Part model, mm, in its own coordinate system. Face numbers are marked on the shaded views. A direction names the side the tool comes from. Coordinates: 2 decimals unless noted, no trailing zeros. Loops run counter-clockwise (first coordinate to the right, second up) from the corner with the lowest first, then second, coordinate; pieces in that order, holes last. Notation, with made-up numbers: (9.25, 48) -> (21.25, 48) arc R13 cw to (21.25, 59) -> close; hole circle Ø8 at (19, 68). An arc over 180 degrees is marked (long way). Use one line per item in the form item = value. Start each with the question number.
(1) Drill centre lines: L1, parallel to X at y = 39, z = 5.25; L2, parallel to Y at x = 0.25, z = 2.5; L3, parallel to Z at x = 8.25, y = -20.5. Where is each one in solid material? Low to high. Write a range as [from, to].
(2) Pin check, flat tips, straight feed: P1, Ø5, axis at x = -9.39, y = 0.55, coming from the +Z side; P2, Ø5, axis at x = 1.5, z = 11.5, coming from the -Y side; P3, Ø5, axis at x = -9.5, z = 17.5, coming from the -Y side; P4, Ø3, axis at x = 6.91, z = 10, coming from the +Y side. Stop position of each tip, or through.
(3) Band-saw the part on B-B on y = 15. Give the cut face in (x, z), then the cut area to 3 significant figures.
(4) Band-saw the part on A-A on y = -31.5. Give the cut face in (x, z) (3 decimals), then the cut area to 3 significant figures.
(5) 3-axis set-ups, long thin cutter, end or side, ignore diameter. For the marked faces 1 and 2: which of +Z, -Z, +X, -X, +Y, -Y reach the whole face in a straight line?
(6) Band-saw the part on C-C on z = 10.75. Count the separate pieces of the cut face and the enclosed holes in it, then the cut area to 3 significant figures.
(7) Mould opens along X. For the marked faces 3, 4 and 5 say: +X half, -X half, draft (parallel to the pull), parting line (faces both ways), or undercut.
```python
from build123d import *

# Parameters (mm, degrees)
ESQUISSE1_W                  = 22.45
ESQUISSE1_H                  = 85
BOSS_EXTRU_1_DEPTH           = 4
ESQUISSE2_R                  = 3
ENL_V_MAT_EXTRU_1_DEPTH      = 4
ESQUISSE3_R                  = 1.6
ENL_V_MAT_EXTRU_2_DEPTH      = 4
ESQUISSE4_W                  = 3
ESQUISSE4_H                  = 38.437504141
BOSS_EXTRU_2_DEPTH           = 20
CONG_1_R                     = 2
ESQUISSE7_W                  = 27.642878523
ESQUISSE7_H                  = 19.995510754
BOSS_EXTRU_3_DEPTH           = 2
BOSS_EXTRU_3_TAPER           = 1
BOSS_EXTRU_3_OTHER_WAY_DEPTH = 1
BOSS_EXTRU_3_OTHER_WAY_TAPER = 1
ESQUISSE8_R                  = 1.7
ENL_V_MAT_EXTRU_3_DEPTH      = 58


with BuildPart() as part:
    # Esquisse1 → Boss.-Extru.1 (new body)
    with BuildSketch(Plane.XY):
        Rectangle(ESQUISSE1_W, ESQUISSE1_H)
    extrude(amount=BOSS_EXTRU_1_DEPTH)

    # Esquisse2 → Enlèv. mat.-Extru.1 (cut)
    with BuildSketch(Plane.XY):
        with Locations((0, -31.5)):
            Circle(ESQUISSE2_R)
    extrude(amount=ENL_V_MAT_EXTRU_1_DEPTH, mode=Mode.SUBTRACT)

    # Esquisse3 → Enlèv. mat.-Extru.2 (cut)
    with BuildSketch(Plane.XY):
        with Locations((-9.391474789, 0.549780329)):
            Circle(ESQUISSE3_R)
        with Locations((9.359403649, 0.04974993)):
            Circle(ESQUISSE3_R)
    extrude(amount=ENL_V_MAT_EXTRU_2_DEPTH, mode=Mode.SUBTRACT)

    # Esquisse4 → Boss.-Extru.2 (add)
    with BuildSketch(Plane.XY):
        with Locations((12.325615706, 23.28124793)):
            Rectangle(ESQUISSE4_W, ESQUISSE4_H)
        with Locations((-12.317262817, 23.407822495)):
            Rectangle(ESQUISSE4_W, ESQUISSE4_H)
    extrude(amount=BOSS_EXTRU_2_DEPTH)

    # Congé1
    cong_1_edges = [part.edges().sort_by_distance(p)[0] for p in [
        (13.825615706, 4.062495859, 10),
        (-13.817262817, 4.189070425, 10),
        (-11.225, -42.5, 2),
        (11.225, -42.5, 2),
    ]]
    fillet(cong_1_edges, radius=CONG_1_R)

    # Esquisse7 → Boss.-Extru.3 (add)
    with BuildSketch(Plane(origin=(0, 42.5, 0), x_dir=(1, 0, 0), z_dir=(0, 1, 0))):
        with Locations((0.004176444, -9.997755377)):
            Rectangle(ESQUISSE7_W, ESQUISSE7_H)
    extrude(amount=BOSS_EXTRU_3_DEPTH, taper=BOSS_EXTRU_3_TAPER)

    # Esquisse7 → Boss.-Extru.3 other way (add)
    with BuildSketch(Plane(origin=(0, 42.5, 0), x_dir=(1, 0, 0), z_dir=(0, 1, 0))):
        with Locations((0.004176444, -9.997755377)):
            Rectangle(ESQUISSE7_W, ESQUISSE7_H)
    extrude(amount=-BOSS_EXTRU_3_OTHER_WAY_DEPTH, taper=BOSS_EXTRU_3_OTHER_WAY_TAPER)

    # Esquisse8 → Enlèv. mat.-Extru.3 (cut)
    with BuildSketch(Plane(origin=(0, 0, 0), x_dir=(1, 0, 0), z_dir=(0, 1, 0))):
        with Locations((6.913641528, -9.997755377)):
            Circle(ESQUISSE8_R)
        with Locations((-7.178390026, -9.997755377)):
            Circle(ESQUISSE8_R)
    extrude(amount=ENL_V_MAT_EXTRU_3_DEPTH, mode=Mode.SUBTRACT)


solid = part.part
```
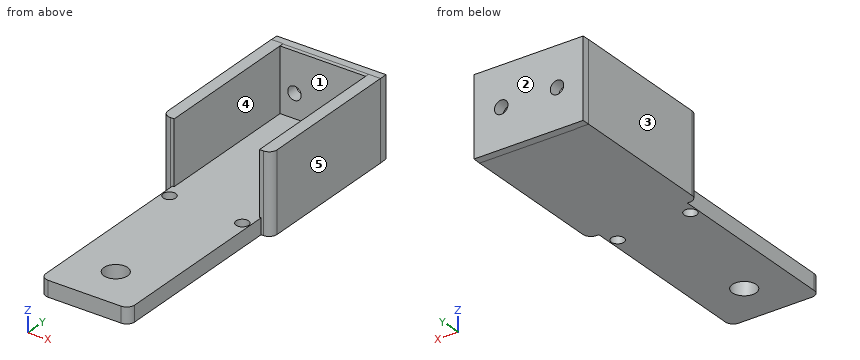
A:
q1.L1 = [-13.82, -10.82], [10.83, 13.83]
q1.L2 = [-42.5, -34.49], [-28.51, 44.5]
q1.L3 = [0, 4]
q2.P1 = 4
q2.P2 = 41.5
q2.P3 = 4.19
q2.P4 = through
q3.outline = (-13.82, 0) -> (13.83, 0) -> (13.83, 20) -> (10.83, 20) -> (10.83, 4) -> (-10.82, 4) -> (-10.82, 20) -> (-13.82, 20) -> close
q3.area = 207 mm²
q4.outline = (-11.225, 0) -> (-3, 0) -> (-3, 4) -> (-11.225, 4) -> close; (3, 0) -> (11.225, 0) -> (11.225, 4) -> (3, 4) -> close
q4.area = 65.8 mm²
q5.face_1 = +Z, -Y
q5.face_2 = +Z, -Z, +X, -X, +Y
q6.separate_pieces = 3
q6.enclosed_holes = 0
q6.area = 287 mm²
q7.face_3 = -X half
q7.face_4 = undercut
q7.face_5 = +X half
